Here's how the part is built. I have some questions about the finished solid (model axes, mm). A direction names the side the tool comes from. Coordinates: 2 decimals unless noted, no trailing zeros. Order: outer loops, then holes, each group sorted by start corner. A loop starts at its lowest first (then second) coordinate and runs counter-clockwise, first axis right, second up. Notation, with made-up numbers: (21.5, 28.25) - (45.5, 28.25) arc R30 cw to (45.5, 52.25) - close; hole circle Ø9 at (0, 21.5). An arc over 180 degrees is marked (long way). Use CSV: the item, a comma, the result in double quotes. Start each with the question number.
from build123d import *

# Parameters (mm, degrees)
SKETCH_3_W          = 170
SKETCH_3_H          = 128
EXTRUDE_2_DEPTH     = 2
SKETCH_4_W          = 166
SKETCH_4_H          = 125
EXTRUDE_3_DEPTH     = 5
CUT_EXTRUDE_1_DEPTH = 5
SKETCH_7_W          = 70
SKETCH_7_H          = 10
CUT_EXTRUDE_3_DEPTH = 107.517604179
SKETCH_6_W          = 4
SKETCH_6_H          = 4
CUT_EXTRUDE_4_DEPTH = 107.630202101


with BuildPart() as part:
    # 草图3 → 凸台-拉伸2 (new body)
    with BuildSketch(Plane.XY):
        Rectangle(SKETCH_3_W, SKETCH_3_H)
    extrude(amount=EXTRUDE_2_DEPTH)

    # 草图4 → 凸台-拉伸3 (add)
    with BuildSketch(Plane.XY.offset(2)):
        Rectangle(SKETCH_4_W, SKETCH_4_H)
    extrude(amount=EXTRUDE_3_DEPTH)

    # 草图5 → 切除-拉伸1 (cut)
    with BuildSketch(Plane.XY.offset(7)):
        Polygon((-80.5, 60), (80.5, 60), (80.5, 52.5), (83, 52.5), (83, 7.5), (80.5, 7.5), (80.5, -60), (-80.5, -60), align=None)
    extrude(amount=-CUT_EXTRUDE_1_DEPTH, mode=Mode.SUBTRACT)

    # 草图7 → 切除-拉伸3 (cut, through all)
    with BuildSketch(Plane.XY.offset(2)):
        with Locations((-40, -50.337089846)):
            Rectangle(SKETCH_7_W, SKETCH_7_H)
        with Locations((40, -50.337089846)):
            Rectangle(SKETCH_7_W, SKETCH_7_H)
        with Locations((-40, -30.337089846)):
            Rectangle(SKETCH_7_W, SKETCH_7_H)
        with Locations((40, -30.337089846)):
            Rectangle(SKETCH_7_W, SKETCH_7_H)
        with Locations((-40, -10.337089846)):
            Rectangle(SKETCH_7_W, SKETCH_7_H)
        with Locations((40, -10.337089846)):
            Rectangle(SKETCH_7_W, SKETCH_7_H)
        with Locations((-40, 9.662910154)):
            Rectangle(SKETCH_7_W, SKETCH_7_H)
        with Locations((40, 9.662910154)):
            Rectangle(SKETCH_7_W, SKETCH_7_H)
        with Locations((-40, 49.662910154)):
            Rectangle(SKETCH_7_W, SKETCH_7_H)
        with Locations((40, 49.662910154)):
            Rectangle(SKETCH_7_W, SKETCH_7_H)
    extrude(amount=-CUT_EXTRUDE_3_DEPTH, mode=Mode.SUBTRACT)

    # 草图6 → 切除-拉伸4 (cut, through all)
    with BuildSketch(Plane(origin=(0, 0, 0), x_dir=(-1, 0, 0), z_dir=(0, 0, -1))):
        with Locations((-78.5, 39.93)):
            Rectangle(SKETCH_6_W, SKETCH_6_H)
        with Locations((78.5, 39.93)):
            Rectangle(SKETCH_6_W, SKETCH_6_H)
    extrude(amount=-CUT_EXTRUDE_4_DEPTH, mode=Mode.SUBTRACT)


solid = part.part
Item 1: We'd pull the mould along X, two halves only. Please class faces 1 (the flat face through (-0.4, 60.5, 7)), 2 (the flat face through (-1, 1, 2)), 3 (the flat face through (83, -28, 4)), 4 (the flat face through (-83, -1, 4)): released by +X, released by -X, zero draft, split by the parting line, or undercut.
Item 2: For pin 1 Ø1 at (x, y) = (-22, 32) entering from -Z; pin 2 Ø1 at (y, z) = (-32, 4) entering from +X; pin 3 Ø2.5 at (y, z) = (4.5, 5.5) entering from -X; pin 4 Ø1.5 at (x, z) = (67, 4) entering from +Y, each with a flat end and sliding along its axis, tell me the tip position at first contact or that it passes through.
Item 3: Suppose I cut it at B-B on y = -53. Write out the boundary of the cut face in (x, z), then the cut area to 3 significant figures.
Item 4: Suppose I cut it at D-D on y = -21. Write out the boundary of the cut face in (x, z), then the cut area to 3 significant figures.
Item 5: Suppose I cut it at A-A on x = -12. State how many separate pieces and enclosed holes the cut face has, then the cut area to 3 significant figures.
Item 6: For faces 5 (the flat face through (83, 57, 4)), 6 (the flat face through (-1, -62.5, 4)), 7 (the flat face through (80.5, 56, 5)), which set-ups out of +Z, -Z, +X, -X, +Y, -Y let a thin tool reach every point of the face, with its end or its side?
Item 7: Please list where these lines run through material, in increasing order: line 1 along Y through (x, z) = (-65, 1.25); line 2 along X through (y, z) = (-31.5, 1.5); line 3 along X through (y, z) = (39, 1.5). Write a range as from..to.
Item 8: Suppose I cut it at C-C on z = 4.5. Write out the boundary of the cut face in (x, y), then the cut area to 3 significant figures.
Here are the results:
1,face 1,"zero draft"
1,face 2,"undercut"
1,face 3,"released by +X"
1,face 4,"released by -X"
2,pin 1,"z = 0"
2,pin 2,"x = 83"
2,pin 3,"x = -83"
2,pin 4,"y = 62.5"
3,outline,"(-85, 0) - (-75, 0) - (-75, 2) - (-80.5, 2) - (-80.5, 7) - (-83, 7) - (-83, 2) - (-85, 2) - close; (-5, 0) - (5, 0) - (5, 2) - (-5, 2) - close; (75, 0) - (85, 0) - (85, 2) - (83, 2) - (83, 7) - (80.5, 7) - (80.5, 2) - (75, 2) - close"
3,area,"85.0 mm^2"
4,outline,"(-85, 0) - (85, 0) - (85, 2) - (83, 2) - (83, 7) - (80.5, 7) - (80.5, 2) - (-80.5, 2) - (-80.5, 7) - (-83, 7) - (-83, 2) - (-85, 2) - close"
4,area,"365 mm^2"
5,separate pieces,"6"
5,enclosed holes,"0"
5,area,"181 mm^2"
6,face 5,"+Z, +X, +Y, -Y"
6,face 6,"+Z, +X, -X, -Y"
6,face 7,"+Z"
7,line 1,"-64..-55.34, -45.34..-35.34, -25.34..-15.34, -5.34..4.66, 14.66..44.66, 54.66..64"
7,line 2,"-85..-75, -5..5, 75..85"
7,line 3,"-85..-80.5, -76.5..76.5, 80.5..85"
8,outline,"(-83, -62.5) - (83, -62.5) - (83, 7.5) - (80.5, 7.5) - (80.5, -60) - (-80.5, -60) - (-80.5, 60) - (80.5, 60) - (80.5, 52.5) - (83, 52.5) - (83, 62.5) - (-83, 62.5) - close"
8,area,"1,320 mm^2"
